Autodesk Inventor part; units mm, degrees
ref_plane "YZ Plane" through (0, 0, 0) normal (1, 0, 0) x (0, 1, 0)
ref_plane "XZ Plane" through (0, 0, 0) normal (0, 1, 0) x (-1, 0, 0)
ref_plane "XY Plane" through (0, 0, 0) normal (0, 0, 1) x (1, 0, 0)
sketch "スケッチ1" plane through (0, 0, 0) normal (0, 0, 1) x (1, 0, 0)
  line L0 (5, -2.5) -> (-5, -2.5)
  line L1 (-5, -2.5) -> (-5, 2.5)
  line L2 (-5, 2.5) -> (5, 2.5)
  line L3 (5, 2.5) -> (5, -2.5)
  line L4 (5, -2.5) -> (-5, 2.5) construction
  line L5 (-5, -2.5) -> (5, 2.5) construction
  circle A0 centre (-3, -0.5) radius 1.15
  circle A1 centre (3, -0.5) radius 1.15
  point P0 (0, 0)
  dimension "d0" = 10
  dimension "d1" = 5
  dimension "d2" = 2.3
  dimension "d3" = 2.3
extrude "押し出し1" add sketch "スケッチ1" along normal blind 4
sketch "スケッチ2" plane through (0, 0, 4) normal (0, 0, 1) x (1, 0, 0)
  circle A0 centre (-3, -0.5) radius 1.15
  circle A1 centre (-3, -0.5) radius 1.9
  circle A2 centre (3, -0.5) radius 1.15
  circle A3 centre (3, -0.5) radius 1.9
  point P0 (0, 0)
  dimension "d6" = 3.8
  dimension "d7" = 3.8
extrude "押し出し2" cut sketch "スケッチ2" against normal blind 2
sketch "スケッチ3" plane through (-5, -2.5, 0) normal (0, -1, 0) x (1, 0, 0)
  line L0 (10, 0) -> (0, 0)
  line L1 (0, 0) -> (10, 0)
  line L2 (10, 0) -> (10, 4)
  line L3 (10, 4) -> (0, 4)
  line L4 (0, 4) -> (0, 0)
  point P0 (5, 0)
extrude "押し出し3" add sketch "スケッチ3" along normal blind 0.5
sketch "スケッチ4" plane through (-5, 2.5, 0) normal (-1, 0, 0) x (0, 0, 1)
  line L0 (0, 0) -> (0, -5.5)
  line L1 (0, 0) -> (4, 0)
  line L2 (0, -5.5) -> (4, -5.5)
  line L3 (4, -5.5) -> (4, 0)
  line L4 (4, 0) -> (0, 0)
  line L5 (0, 0) -> (0, -5.5)
  point P0 (0, -2.5)
extrude "押し出し4" add sketch "スケッチ4" along normal blind 0.5
sketch "スケッチ5" plane through (5, 2.5, 4) normal (1, 0, 0) x (0, 0, -1)
  line L0 (4, 0) -> (4, -5.5)
  line L1 (4, 0) -> (0, 0)
  line L2 (4, -5.5) -> (0, -5.5)
  line L3 (0, -5.5) -> (0, 0)
  line L4 (0, 0) -> (4, 0)
  line L5 (4, 0) -> (4, -5.5)
  point P0 (4, -2.5)
extrude "押し出し5" add sketch "スケッチ5" along normal blind 0.5
sketch "スケッチ6" plane through (0, 0, 4) normal (0, 0, 1) x (1, 0, 0)
  line L0 (-5.5, 2.5) -> (5.5, 2.5)
  line L1 (-5.5, 2.5) -> (5.5, 2.5)
  line L2 (5.5, 2.5) -> (5.5, -3)
  line L3 (5.5, 2.5) -> (5.5, 2.2)
  line L4 (5.5, 2.2) -> (-5.5, 2.2)
  line L5 (-5.5, -3) -> (-5.5, 2.5)
  line L6 (-5.5, 2.2) -> (-5.5, 2.5)
  line L7 (-5.5, 2.2) -> (-5.3268, 2.5)
  line L8 (-5.5, 2.2) -> (-5.1536, 2.2) construction
  line L9 (-5.3268, 2.5) -> (-5.1536, 2.2)
  line L10 (-5.1536, 2.2) -> (-4.9804, 2.5)
  line L11 (-4.9804, 2.5) -> (-4.8072, 2.2)
  line L12 (-4.8072, 2.2) -> (-4.634, 2.5)
  line L13 (-4.634, 2.5) -> (-4.4608, 2.2)
  line L14 (-4.4608, 2.2) -> (-4.2876, 2.5)
  line L15 (-4.2876, 2.5) -> (-4.1144, 2.2)
  line L16 (-4.1144, 2.2) -> (-3.9412, 2.5)
  line L17 (-3.9412, 2.5) -> (-3.7679, 2.2)
  line L18 (-3.7679, 2.2) -> (-3.5947, 2.5)
  line L19 (-3.5947, 2.5) -> (-3.4215, 2.2)
  line L20 (-3.4215, 2.2) -> (-3.2483, 2.5)
  line L21 (-3.2483, 2.5) -> (-3.0751, 2.2)
  line L22 (-3.0751, 2.2) -> (-2.9019, 2.5)
  line L23 (-2.9019, 2.5) -> (-2.7287, 2.2)
  line L24 (-2.7287, 2.2) -> (-2.5869, 2.5)
  line L25 (-2.5869, 2.5) -> (-2.4137, 2.2)
  line L26 (-2.4137, 2.2) -> (-2.2405, 2.5)
  line L27 (-2.2405, 2.5) -> (-2.0673, 2.2)
  line L28 (-2.0673, 2.2) -> (-1.8941, 2.5)
  line L29 (-1.8941, 2.5) -> (-1.7209, 2.2)
  line L30 (-1.7209, 2.2) -> (-1.5477, 2.5)
  line L31 (-1.5477, 2.5) -> (-1.3745, 2.2)
  line L32 (-1.3745, 2.2) -> (-1.2012, 2.5)
  line L33 (-1.2012, 2.5) -> (-1.028, 2.2)
  line L34 (-1.028, 2.2) -> (-0.8548, 2.5)
  line L35 (-0.8548, 2.5) -> (-0.6816, 2.2)
  line L36 (-0.6816, 2.2) -> (-0.5084, 2.5)
  line L37 (-0.5084, 2.5) -> (-0.3352, 2.2)
  line L38 (-0.3352, 2.2) -> (-0.162, 2.5)
  line L39 (-0.162, 2.5) -> (0.0112, 2.2)
  line L40 (0.0112, 2.2) -> (0.1844, 2.5)
  line L41 (0.1844, 2.5) -> (0.3576, 2.2)
  line L42 (0.3576, 2.2) -> (0.5308, 2.5)
  line L43 (0.5308, 2.5) -> (0.704, 2.2)
  line L44 (0.704, 2.2) -> (0.8772, 2.5)
  line L45 (0.8772, 2.5) -> (1.0504, 2.2)
  line L46 (1.0504, 2.2) -> (1.2236, 2.5)
  line L47 (1.2236, 2.5) -> (1.3968, 2.2)
  line L48 (1.3968, 2.2) -> (1.57, 2.5)
  line L49 (1.57, 2.5) -> (1.7432, 2.2)
  line L50 (1.7432, 2.2) -> (1.9164, 2.5)
  line L51 (1.9164, 2.5) -> (2.0897, 2.2)
  line L52 (2.0897, 2.2) -> (2.2629, 2.5)
  line L53 (2.2629, 2.5) -> (2.4361, 2.2)
  line L54 (2.4361, 2.2) -> (2.6093, 2.5)
  line L55 (2.6093, 2.5) -> (2.7825, 2.2)
  line L56 (2.7825, 2.2) -> (2.9557, 2.5)
  line L57 (2.9557, 2.5) -> (3.1289, 2.2)
  line L58 (3.1289, 2.2) -> (3.3021, 2.5)
  line L59 (3.3021, 2.5) -> (3.4753, 2.2)
  line L60 (3.4753, 2.2) -> (3.6485, 2.5)
  line L61 (3.6485, 2.5) -> (3.8217, 2.2)
  line L62 (3.8217, 2.2) -> (3.9949, 2.5)
  line L63 (3.9949, 2.5) -> (4.1681, 2.2)
  line L64 (4.1681, 2.2) -> (4.3413, 2.5)
  line L65 (4.3413, 2.5) -> (4.5145, 2.2)
  line L66 (4.5145, 2.2) -> (4.6877, 2.5)
  line L67 (4.6877, 2.5) -> (4.8609, 2.2)
  line L68 (4.8609, 2.2) -> (5.0341, 2.5)
  line L69 (5.0341, 2.5) -> (5.2073, 2.2)
  line L70 (5.2073, 2.2) -> (5.3805, 2.5)
  line L71 (5.3805, 2.5) -> (5.5, 2.2)
  point P0 (0, 0)
  dimension "d16" = 0.3
  dimension "d17" = 60
extrude "押し出し6" cut sketch "スケッチ6" against normal blind 10 contours L0 L7 L5 | L0 L10 L9 | L0 L12 L11 | L0 L14 L13 | L0 L16 L15 | L0 L18 L17 | L0 L20 L19 | L0 L22 L21 | L0 L24 L23 | L0 L26 L25 | L0 L28 L27 | L0 L30 L29 | L0 L32 L31 | L0 L34 L33 | L0 L36 L35 | L0 L38 L37 | L0 L40 L39 | L0 L42 L41 | L0 L44 L43 | L0 L46 L45 | L0 L48 L47 | L0 L50 L49 | L0 L52 L51 | L0 L54 L53 | L0 L56 L55 | L0 L58 L57 | L0 L60 L59 | L0 L62 L61 | L0 L64 L63 | L0 L66 L65 | L0 L68 L67 | L0 L70 L69 | L0 L2 L71
properties part number "gripping_base" material "ゴム、黒"
The listing builds one solid part. Answer for the finished solid, in the listing's coordinates (mm). A direction names the side the tool comes from. Round coordinates to 2 decimals unless told otherwise and drop trailing zeros. Loops run counter-clockwise (first coordinate to the right, second up) from the corner with the lowest first, then second, coordinate; pieces in that order, holes last. Notation, with made-up numbers: (-32, 25) - (-15, 25) arc R30 cw to (-15, 50) - close; hole circle Ø1 at (47, -34.75). An arc over 180 degrees is marked (long way). Return JSON: item names as keys, results as strings. Group by question number.
1. Which of the six approach directions +Z, -Z, +X, -X, +Y, -Y give full straight-line access (tool end or side, diameter ignored) to faces 1 (the flat face through (-3, -2, 2)), 2 (the cylindrical face through (-1.938, -0.06, 0.986))?
2. The part is cut by section A-A on y = -0.5. Determine the outline of the cut face in (x, z).
3. Consider probe 1 along Z at (x, y) = (-3, -1.8); probe 2 along X at (y, z) = (-1.45, 3.05); probe 3 along Y at (x, z) = (-3, 1.6). Determine where each line is inside the solid, lowest interval first.
4. The part is cut by section B-B on z = 1.25. State how many separate pieces and enclosed holes the cut face has, then the cut area to 3 significant figures.
5. The mould has two halves that part along X. Classify faces 3 (the flat face through (-5.5, 0, 2)), 4 (the cylindrical face through (-3.412, -2.355, 3.014)), 5 (the flat face through (5.5, 0, 2)): pulls with the +X half, pulls with the -X half, needs draft (parallel to the pull), parting line crosses it, or undercut.
Resolved:
{
 "1": {"face 1": "+Z", "face 2": "+Z, -Z"},
 "2": {"outline": "(-5.5, 0) - (-4.15, 0) - (-4.15, 2) - (-4.9, 2) - (-4.9, 4) - (-5.5, 4) - close; (-1.85, 0) - (1.85, 0) - (1.85, 2) - (1.1, 2) - (1.1, 4) - (-1.1, 4) - (-1.1, 2) - (-1.85, 2) - close; (4.15, 0) - (5.5, 0) - (5.5, 4) - (4.9, 4) - (4.9, 2) - (4.15, 2) - close"},
 "3": {"probe 1": "z = 0 to 2", "probe 2": "x = -5.5 to -4.65, -1.35 to 1.35, 4.65 to 5.5", "probe 3": "y = -3 to -1.65, 0.65 to 2.33"},
 "4": {"separate pieces": "1", "enclosed holes": "2", "area": "50.5 mm²"},
 "5": {"face 3": "pulls with the -X half", "face 4": "undercut", "face 5": "pulls with the +X half"}
}
